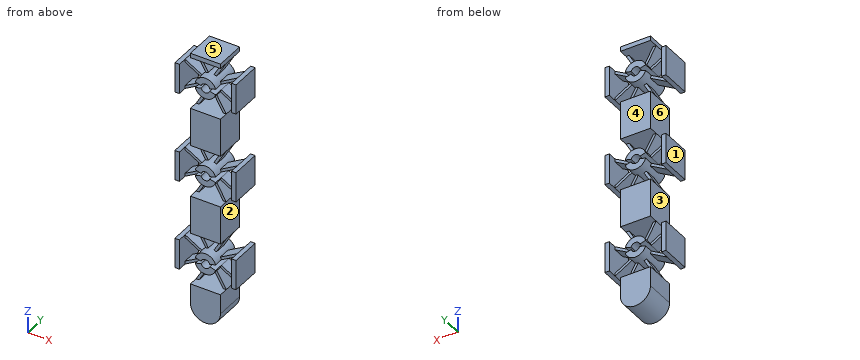
from build123d import *

# Parameters (mm, degrees)
SKETCH1_W                     = 10
SKETCH1_H                     = 1.5
BASE_BUTTERFLY_BLOCKS_DEPTH   = 5
SKETCH1_W_2                   = 1.5
SKETCH1_H_2                   = 10
BASE_BUTTERFLY_BLOCKS_2_DEPTH = 5
BASE_BUTTERFLY_BLOCKS_3_DEPTH = 5
BASE_BUTTERFLY_BLOCKS_4_DEPTH = 5
BASE_BUTTERFLY_BLOCKS_5_DEPTH = 5
BASE_BUTTERFLY_BLOCKS_6_DEPTH = 5
BASE_BUTTERFLY_FLEXURES_DEPTH = 2
LPATTERN1_COUNT               = 3
LPATTERN1_PITCH               = 30
SKETCH3_W                     = 10
SKETCH3_H                     = 10
PIP_DEPTH                     = 9.679491924
SKETCH5_W                     = 10
SKETCH5_H                     = 10
BOSS_EXTRUDE7_DEPTH           = 9.679491924
SKETCH6_W                     = 10
SKETCH6_H                     = 5
BOSS_EXTRUDE9_DEPTH           = 10


with BuildPart() as part:
    # Sketch1 → base_butterfly_blocks (new, symmetric)
    with BuildSketch(Plane(origin=(0, 0, 0), x_dir=(1, 0, 0), z_dir=(0, 1, 0))):
        with Locations((0, -9.410254038)):
            Rectangle(SKETCH1_W, SKETCH1_H)
    extrude(amount=BASE_BUTTERFLY_BLOCKS_DEPTH, both=True)



with BuildPart() as body_2:
    # Sketch1 → base_butterfly_blocks 2 (new, symmetric)
    with BuildSketch(Plane(origin=(0, 0, 0), x_dir=(1, 0, 0), z_dir=(0, 1, 0))):
        with Locations((-9.410254038, 0)):
            Rectangle(SKETCH1_W_2, SKETCH1_H_2)
    extrude(amount=BASE_BUTTERFLY_BLOCKS_2_DEPTH, both=True)


with BuildPart() as body_3:
    # Sketch1 → base_butterfly_blocks 3 (new, symmetric)
    with BuildSketch(Plane(origin=(0, 0, 0), x_dir=(1, 0, 0), z_dir=(0, 1, 0))):
        with Locations((0, 9.410254038)):
            Rectangle(SKETCH1_W, SKETCH1_H)
    extrude(amount=BASE_BUTTERFLY_BLOCKS_3_DEPTH, both=True)


with BuildPart() as body_4:
    # Sketch1 → base_butterfly_blocks 4 (new, symmetric)
    with BuildSketch(Plane(origin=(0, 0, 0), x_dir=(1, 0, 0), z_dir=(0, 1, 0))):
        with Locations((9.410254038, 0)):
            Rectangle(SKETCH1_W_2, SKETCH1_H_2)
    extrude(amount=BASE_BUTTERFLY_BLOCKS_4_DEPTH, both=True)


with BuildPart() as body_5:
    # Sketch1 → base_butterfly_blocks 5 (new, symmetric)
    with BuildSketch(Plane(origin=(0, 0, 0), x_dir=(1, 0, 0), z_dir=(0, 1, 0))):
        with BuildLine():
            Line((-1.444220457, 0.405249641), (-3.369847733, 0.945582496))
            ThreePointArc((-3.369847733, 0.945582496), (0, 3.5), (3.369847733, 0.945582496))
            Line((3.369847733, 0.945582496), (1.444220457, 0.405249641))
            ThreePointArc((1.444220457, 0.405249641), (0, 1.5), (-1.444220457, 0.405249641))
        make_face()
    extrude(amount=BASE_BUTTERFLY_BLOCKS_5_DEPTH, both=True)


with BuildPart() as body_6:
    # Sketch1 → base_butterfly_blocks 6 (new, symmetric)
    with BuildSketch(Plane(origin=(0, 0, 0), x_dir=(1, 0, 0), z_dir=(0, 1, 0))):
        with BuildLine():
            ThreePointArc((-1.444220457, -0.405249641), (0, -1.5), (1.444220457, -0.405249641))
            Line((1.444220457, -0.405249641), (3.369847733, -0.945582496))
            ThreePointArc((3.369847733, -0.945582496), (0, -3.5), (-3.369847733, -0.945582496))
            Line((-3.369847733, -0.945582496), (-1.444220457, -0.405249641))
        make_face()
    extrude(amount=BASE_BUTTERFLY_BLOCKS_6_DEPTH, both=True)


with BuildPart() as part_1:
    add(part.part)

    add(body_2.part)  # base_butterfly_flexures merges body 2

    add(body_3.part)  # base_butterfly_flexures merges body 3

    add(body_4.part)  # base_butterfly_flexures merges body 4

    add(body_5.part)  # base_butterfly_flexures merges body 5

    add(body_6.part)  # base_butterfly_flexures merges body 6
    # Sketch1<4> → base_butterfly_flexures (add, symmetric)
    with BuildSketch(Plane(origin=(0, 0, 0), x_dir=(1, 0, 0), z_dir=(0, 1, 0))):
        with BuildLine():
            Line((-8.660254038, 5), (-8.660254038, 4))
            Line((-8.660254038, 4), (-3.369847733, 0.945582496))
            ThreePointArc((-3.369847733, 0.945582496), (-3.225642474, 1.358392665), (-3.031088913, 1.75))
            Line((-3.031088913, 1.75), (-8.660254038, 5))
        make_face()
        with BuildLine():
            Line((-5, 8.660254038), (-1.75, 3.031088913))
            ThreePointArc((-1.75, 3.031088913), (-1.358392665, 3.225642474), (-0.945582496, 3.369847733))
            Line((-0.945582496, 3.369847733), (-4, 8.660254038))
            Line((-4, 8.660254038), (-5, 8.660254038))
        make_face()
        with BuildLine():
            Line((4, 8.660254038), (0.945582496, 3.369847733))
            ThreePointArc((0.945582496, 3.369847733), (1.358392665, 3.225642474), (1.75, 3.031088913))
            Line((1.75, 3.031088913), (5, 8.660254038))
            Line((5, 8.660254038), (4, 8.660254038))
        make_face()
        with BuildLine():
            Line((3.369847733, 0.945582496), (8.660254038, 4))
            Line((8.660254038, 4), (8.660254038, 5))
            Line((8.660254038, 5), (3.031088913, 1.75))
            ThreePointArc((3.031088913, 1.75), (3.225642474, 1.358392665), (3.369847733, 0.945582496))
        make_face()
        with BuildLine():
            ThreePointArc((3.369847733, -0.945582496), (3.225642474, -1.358392665), (3.031088913, -1.75))
            Line((3.031088913, -1.75), (8.660254038, -5))
            Line((8.660254038, -5), (8.660254038, -4))
            Line((8.660254038, -4), (3.369847733, -0.945582496))
        make_face()
        with BuildLine():
            ThreePointArc((1.75, -3.031088913), (1.358392665, -3.225642474), (0.945582496, -3.369847733))
            Line((0.945582496, -3.369847733), (4, -8.660254038))
            Line((4, -8.660254038), (5, -8.660254038))
            Line((5, -8.660254038), (1.75, -3.031088913))
        make_face()
        with BuildLine():
            ThreePointArc((-0.945582496, -3.369847733), (-1.358392665, -3.225642474), (-1.75, -3.031088913))
            Line((-1.75, -3.031088913), (-5, -8.660254038))
            Line((-5, -8.660254038), (-4, -8.660254038))
            Line((-4, -8.660254038), (-0.945582496, -3.369847733))
        make_face()
        with BuildLine():
            Line((-8.660254038, -5), (-3.031088913, -1.75))
            ThreePointArc((-3.031088913, -1.75), (-3.225642474, -1.358392665), (-3.369847733, -0.945582496))
            Line((-3.369847733, -0.945582496), (-8.660254038, -4))
            Line((-8.660254038, -4), (-8.660254038, -5))
        make_face()
    extrude(amount=BASE_BUTTERFLY_FLEXURES_DEPTH, both=True)


with BuildPart() as lpattern1_1:
    # LPattern1: pattern copy
    add(part_1.part.moved(Location(Vector(0, 0, -1) * (1 * LPATTERN1_PITCH))))


with BuildPart() as lpattern1_2:
    # LPattern1: pattern copy
    add(part_1.part.moved(Location(Vector(0, 0, -1) * (2 * LPATTERN1_PITCH))))


with BuildPart() as part_2:
    add(part_1.part)

    add(lpattern1_1.part)  # PIP merges LPattern1_1
    # Sketch3 → PIP (add)
    with BuildSketch(Plane(origin=(0, 0, -10.160254038), x_dir=(-1, 0, 0), z_dir=(0, 0, -1))):
        Rectangle(SKETCH3_W, SKETCH3_H)
    extrude(amount=PIP_DEPTH)

    add(lpattern1_2.part)  # Boss-Extrude7 merges LPattern1_2
    # Sketch5 → Boss-Extrude7 (add)
    with BuildSketch(Plane(origin=(0, 0, -40.160254038), x_dir=(-1, 0, 0), z_dir=(0, 0, -1))):
        Rectangle(SKETCH5_W, SKETCH5_H)
    extrude(amount=BOSS_EXTRUDE7_DEPTH)

    # Sketch6 → Boss-Extrude9 (add)
    with BuildSketch(Plane.XZ.offset(5)):
        with BuildLine():
            Line((-5, -75.160254038), (5, -75.160254038))
            ThreePointArc((5, -75.160254038), (0, -80.160254038), (-5, -75.160254038))
        make_face()
        with Locations((0, -72.660254038)):
            Rectangle(SKETCH6_W, SKETCH6_H)
    extrude(amount=-BOSS_EXTRUDE9_DEPTH)


solid = part_2.part
The listing builds one solid part. Answer for the finished solid, in the listing's coordinates (mm). Face numbers are marked on the shaded views. A direction names the side the tool comes from. Round coordinates to 2 decimals unless told otherwise and drop trailing zeros. Write each loop counter-clockwise with the first axis right and the second up, starting at its lowest first coordinate (ties: lowest second). Pieces come first, ordered by that corner, then holes. Notation, with made-up numbers: M 9,74 L 47,74 A10 cw 47,79 Z; hole C 28.25,0.25 d2. An arc over 180 degrees is marked long. Write each question's results on one line, items separated by ' | '. Start each with the question number.
Item 1: Which of the six approach directions +Z, -Z, +X, -X, +Y, -Y give full straight-line access (tool end or side, diameter ignored) to the marked faces 1, 2 and 3?
Item 2: The mould has two halves that part along Z. Classify the marked faces 4, 5 and 6: +Z half, -Z half, draft (parallel to the pull), parting line (faces both ways), or undercut.
Item 3: Find section C-C on z = -47.5. Write down the section's boundary in (x, y), and give its area (3 significant figures).
Item 4: Straight lines are drawn through the part: probe 1 along X at (y, z) = (2.25, -18); probe 2 along Z at (x, y) = (7, 1.25); probe 3 along Z at (x, y) = (-7.75, -1). For each, find the intervals that lie inside material, in ascending order.
Item 5: Given pin 1 Ø1.6 at (x, y) = (9.5, -1.5) entering from +Z; pin 2 Ø1.2 at (x, z) = (7, -3.5) entering from +Y; pin 3 Ø4.5 at (x, z) = (3, -65.5) entering from -Y, each flat-ended and moving along its own axis, determine where each tip first touches the part or whether it passes through.
Item 6: Find section A-A on x = 0. Give the number of separate pieces and of enclosed holes in the cut face, and give its area (3 significant figures).
Answer block:
1) face 1: +Z, -Z, -X, +Y, -Y | face 2: +X, +Y, -Y | face 3: -X, +Y, -Y
2) face 4: draft | face 5: +Z half | face 6: undercut
3) outline: M -5,-5 L 5,-5 L 5,5 L -5,5 Z | area: 100 mm²
4) probe 1: x = -5 to 5 | probe 2: z = -64.04 to -63.04, -56.96 to -55.96, -34.04 to -33.04, -26.96 to -25.96, -4.04 to -3.04, 3.04 to 4.04 | probe 3: z = -64.47 to -63.47, -56.53 to -55.53, -34.47 to -33.47, -26.53 to -25.53, -4.47 to -3.47, 3.47 to 4.47
5) pin 1: stops at z = 5 | pin 2: stops at y = 2 | pin 3: stops at y = -2
6) separate pieces: 10 | enclosed holes: 0 | area: 504 mm²
